For this review, take the finished solid that the model builds, in its own axes (mm). Face numbers are marked on the shaded views. A direction names the side the tool comes from. Give positions to 0.01 mm unless a question says otherwise; leave off trailing zeros. Write each loop counter-clockwise with the first axis right and the second up, starting at its lowest first coordinate (ties: lowest second). Pieces come first, ordered by that corner, then holes. Notation, with made-up numbers: M 12.5,26.5 L 42.5,26.5 A15 ccw 42.5,36.5 Z; hole C -18.5,-30 d7. An arc over 180 degrees is marked long. Write item = value, one per line.
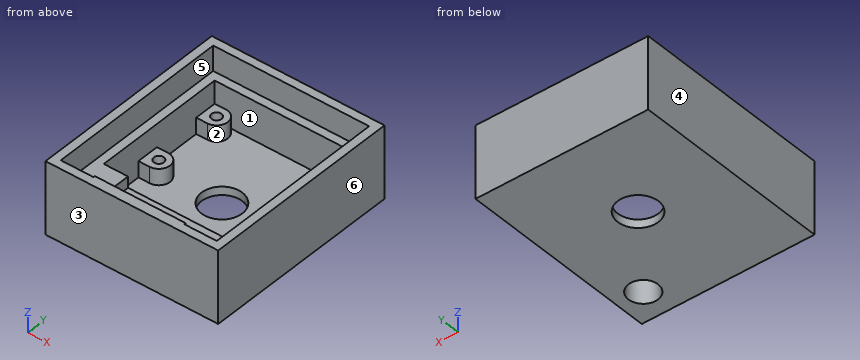
```python
from build123d import *

# Parameters (mm, degrees)
CROQUIS1_W               = 25
CROQUIS1_H               = 24
CROQUIS1_R               = 3.65
SALIENTE_EXTRUIR1_DEPTH  = 1.5
SALIENTE_EXTRUIR7_DEPTH  = 8.5
CROQUIS2_R               = 0.9
SALIENTE_EXTRUIR2_DEPTH  = 2.9
CROQUIS5_W               = 31
CROQUIS5_H               = 9
SALIENTE_EXTRUIR8_DEPTH  = 6.5
CROQUIS6_R               = 2.65
CORTAR_EXTRUIR1_DEPTH    = 6.5
SALIENTE_EXTRUIR9_DEPTH  = 2
CROQUIS8_W               = 31
CROQUIS8_H               = 36
SALIENTE_EXTRUIR10_DEPTH = 4.5
CROQUIS9_W               = 5.85
CROQUIS9_H               = 7.5
CORTAR_EXTRUIR3_DEPTH    = 2


with BuildPart() as part:
    # Croquis1 → Saliente-Extruir1 (new body)
    with BuildSketch(Plane.XY):
        with Locations((0, 1.5)):
            Rectangle(CROQUIS1_W, CROQUIS1_H)
        Circle(CROQUIS1_R, mode=Mode.SUBTRACT)
    extrude(amount=SALIENTE_EXTRUIR1_DEPTH)

    # Croquis4 → Saliente-Extruir7 (add)
    with BuildSketch(Plane(origin=(0, 0, 0), x_dir=(-1, 0, 0), z_dir=(0, 0, -1))):
        Polygon((12.5, -10.5), (12.5, 13.5), (-12.5, 13.5), (-12.5, -10.5), (-15.5, -10.5), (-15.5, 16.5), (15.5, 16.5), (15.5, -10.5), align=None)
    extrude(amount=-SALIENTE_EXTRUIR7_DEPTH)

    # Croquis2 → Saliente-Extruir2 (add)
    with BuildSketch(Plane.XY.offset(1.5)):
        with BuildLine():
            Line((-10.5, 9.5), (-12.5, 9.5))
            Line((-12.5, 9.5), (-12.5, 13.5))
            Line((-12.5, 13.5), (-10.5, 13.5))
            ThreePointArc((-10.5, 13.5), (-8.5, 11.5), (-10.5, 9.5))
        make_face()
        with Locations((-10.5, 11.5)):
            Circle(CROQUIS2_R, mode=Mode.SUBTRACT)
        with BuildLine():
            Line((-10.5, -3), (-12.5, -3))
            Line((-12.5, -3), (-12.5, 1))
            Line((-12.5, 1), (-10.5, 1))
            ThreePointArc((-10.5, 1), (-8.5, -1), (-10.5, -3))
        make_face()
        with Locations((-10.5, -1)):
            Circle(CROQUIS2_R, mode=Mode.SUBTRACT)
    saliente_extruir2 = extrude(amount=SALIENTE_EXTRUIR2_DEPTH)

    # Simetría2: Saliente-Extruir2 across plane
    add(saliente_extruir2.mirror(Plane(origin=(0, 0, 0), x_dir=(0, 0, 1), z_dir=(1, 0, 0))))

    # Croquis5 → Saliente-Extruir8 (add)
    with BuildSketch(Plane(origin=(0, 0, 0), x_dir=(-1, 0, 0), z_dir=(0, 0, -1))):
        with Locations((0, -15)):
            Rectangle(CROQUIS5_W, CROQUIS5_H)
    extrude(amount=-SALIENTE_EXTRUIR8_DEPTH)

    # Croquis6 → Cortar-Extruir1 (cut)
    with BuildSketch(Plane.XY.offset(6.5)):
        with Locations((10.8, -14.15)):
            Circle(CROQUIS6_R)
    extrude(amount=-CORTAR_EXTRUIR1_DEPTH, mode=Mode.SUBTRACT)

    # Croquis7 → Saliente-Extruir9 (add)
    with BuildSketch(Plane.XY.offset(6.5)):
        with BuildLine():
            Line((-15.5, -10.5), (-8.15, -10.5))
            Line((-8.15, -10.5), (-8.15, -17.7))
            Line((-8.15, -17.7), (8.15, -17.7))
            Line((8.15, -17.7), (8.15, -14.768763357))
            Line((8.15, -14.768763357), (8.223251679, -14.768763357))
            ThreePointArc((8.223251679, -14.768763357), (13.448478088, -14.239798753), (8.271080496, -13.35812492))
            Line((8.271080496, -13.35812492), (8.15, -13.35812492))
            Line((8.15, -13.35812492), (8.15, -10.5))
            Line((8.15, -10.5), (15.5, -10.5))
            Line((15.5, -10.5), (15.5, -19.5))
            Line((15.5, -19.5), (8.15, -19.5))
            Line((8.15, -19.5), (-8.15, -19.5))
            Line((-8.15, -19.5), (-15.5, -19.5))
            Line((-15.5, -19.5), (-15.5, -10.5))
        make_face()
    extrude(amount=SALIENTE_EXTRUIR9_DEPTH)

    # Croquis8 → Saliente-Extruir10 (add)
    with BuildSketch(Plane.XY.offset(8.5)):
        with Locations((0, -1.5)):
            Rectangle(CROQUIS8_W, CROQUIS8_H)
        Polygon((-14, 15), (14, 15), (14, -18), (8.15, -18), (8.15, -17.7), (-8.15, -17.7), (-8.15, -18), (-14, -18), align=None, mode=Mode.SUBTRACT)
    extrude(amount=SALIENTE_EXTRUIR10_DEPTH)

    # Croquis9 → Cortar-Extruir3 (cut)
    with BuildSketch(Plane.XY.offset(8.5)):
        with Locations((11.075, -14.25)):
            Rectangle(CROQUIS9_W, CROQUIS9_H)
    extrude(amount=-CORTAR_EXTRUIR3_DEPTH, mode=Mode.SUBTRACT)


solid = part.part
```
1. For line 1 along Y through (x, z) = (11, 6.25); line 2 along Y through (x, z) = (-4, 6.25); line 3 along X through (y, z) = (-9.5, 6.25), list the stretches that pass through material, from the lowest coordinate up. Write a range as from..to.
Responses:
line_1 = -19.5..-16.79, -11.51..-10.5, 13.5..16.5
line_2 = -19.5..-10.5, 13.5..16.5
line_3 = -15.5..-12.5, 12.5..15.5
2. We need section C-C, the plane z = 11.5. Write out the cut boundary in (x, y).
Responses:
outline = M -15.5,-19.5 L 15.5,-19.5 L 15.5,16.5 L -15.5,16.5 Z; hole M -14,-18 L -8.15,-18 L -8.15,-17.7 L 8.15,-17.7 L 8.15,-18 L 14,-18 L 14,15 L -14,15 Z
3. Insertion check: P1, Ø1.4, axis at x = -10.5, y = -0.5, coming from the +Z side; P2, Ø2, axis at x = 1.5, y = -8, coming from the +Z side; P3, Ø4.5, axis at x = -11, y = -1.5, coming from the +Z side. Each pin has a flat end and moves straight along its axis. Give the tip position at first contact, or say it passes through.
Responses:
P1 = 4.4
P2 = 1.5
P3 = 8.5
4. We need section D-D, the plane y = -14.15. Write out the cut boundary in (x, z), then the cut area to 3 significant figures.
Responses:
outline = M -15.5,0 L 8.15,0 L 8.15,6.5 L -8.15,6.5 L -8.15,8.5 L -14,8.5 L -14,13 L -15.5,13 Z; M 13.45,0 L 15.5,0 L 15.5,13 L 14,13 L 14,6.5 L 13.45,6.5 Z
area = 198 mm2
5. The part is to be moulded in two halves that separate along X. For the marked faces 1, 2, 3 and 4, say which applies: +X half, -X half, draft (parallel to the pull), parting line (faces both ways), or undercut.
Responses:
face_1 = undercut
face_2 = undercut
face_3 = draft
face_4 = -X half
6. We need section A-A, the plane x = 0. Write out the cut boundary in (y, z).
Responses:
outline = M -19.5,0 L -3.65,0 L -3.65,1.5 L -10.5,1.5 L -10.5,6.5 L -17.7,6.5 L -17.7,13 L -19.5,13 Z; M 3.65,0 L 16.5,0 L 16.5,13 L 15,13 L 15,8.5 L 13.5,8.5 L 13.5,1.5 L 3.65,1.5 Z
7. Machinability: for the marked faces 5 and 6, which of the approach directions +Z, -Z, +X, -X, +Y, -Y give a long, thin tool a straight path to every point of the face, cutting with its end or side? Answer none if there is none.
Responses:
face_5 = +Z
face_6 = +Z, -Z, +X, +Y, -Y
8. We need section B-B, the plane z = 6. Write out the cut boundary in (x, y), then the cut area to 3 significant figures.
Responses:
outline = M -15.5,-19.5 L 15.5,-19.5 L 15.5,16.5 L -15.5,16.5 Z; hole M -12.5,-10.5 L 12.5,-10.5 L 12.5,13.5 L -12.5,13.5 Z; hole C 10.8,-14.15 d5.3
area = 494 mm2
